Work out the finished part from the listing and answer in its coordinate system (mm). Round coordinates to 2 decimals unless told otherwise and drop trailing zeros. Loops run counter-clockwise (first coordinate to the right, second up) from the corner with the lowest first, then second, coordinate; pieces in that order, holes last. Notation, with made-up numbers: (1, 83.5) - (8, 83.5) arc R15 ccw to (8, 95.5) - close; hole circle Ø7 at (-38, -19.75). An arc over 180 degrees is marked (long way). Answer as CSV lines item,"result". Start each with the question number.
```python
from build123d import *

# Parameters (mm, degrees)
SKETCH1_R           = 1.29
SKETCH1_R_2         = 2
BOSS_EXTRUDE1_DEPTH = 1.5
FILLET1_R           = 2


with BuildPart() as part:
    # Sketch1 → Boss-Extrude1 (new, symmetric)
    with BuildSketch(Plane.XY):
        with BuildLine():
            Line((-9.367496998, 3.5), (30, 3.5))
            ThreePointArc((30, 3.5), (33.5, 0), (30, -3.5))
            Line((30, -3.5), (-9.367496998, -3.5))
            ThreePointArc((-9.367496998, -3.5), (-10, 0), (-9.367496998, 3.5))
        make_face()
        with Locations((-7, 0)):
            Circle(SKETCH1_R, mode=Mode.SUBTRACT)
        with Locations((7, 0)):
            Circle(SKETCH1_R, mode=Mode.SUBTRACT)
        with Locations((30, 0)):
            Circle(SKETCH1_R, mode=Mode.SUBTRACT)
        Circle(SKETCH1_R_2, mode=Mode.SUBTRACT)
    extrude(amount=BOSS_EXTRUDE1_DEPTH, both=True)

    # Fillet1
    fillet1_edges = [part.edges().sort_by_distance(p)[0] for p in [
        (-9.367496998, 3.5, 0),
        (-9.367496998, -3.5, 0),
    ]]
    fillet(fillet1_edges, radius=FILLET1_R)


solid = part.part
```
Item 1: Section A-A, the plane x = 7 is taken. Give the vertices of the cut face in (y, z), and give its area (3 significant figures).
Item 2: Section B-B, the plane z = -0.8 is taken. Give the vertices of the cut face in (x, y) (3 decimals).
Item 3: Determine the mould class of faces 1 (the face through (5.976, -0.785, -0.021)), 2 (the face through (-10, 0, 0)), 3 (the face through (12, 0, -1.5)) for opening direction X: pulls with the +X half, pulls with the -X half, needs draft (parallel to the pull), parting line crosses it, or undercut.
Item 4: Find the intervals of material crossed by L1, parallel to Y at x = -7, z = 0.3; L2, parallel to X at y = -0.75, z = 0.95; L3, parallel to X at y = -1, z = -0.9, in increasing order.
Answer:
1,outline,"(-3.5, -1.5) - (-1.29, -1.5) - (-1.29, 1.5) - (-3.5, 1.5) - close; (1.29, -1.5) - (3.5, -1.5) - (3.5, 1.5) - (1.29, 1.5) - close"
1,area,"13.3 mm²"
2,outline,"(-9.823, -1.875) arc R2 ccw to (-7.858, -3.5) - (30, -3.5) arc R3.5 ccw to (30, 3.5) - (-7.858, 3.5) arc R2 ccw to (-9.823, 1.875) arc R10 ccw to start; hole circle Ø2.58 at (-7, 0); hole circle Ø4 at (0, 0); hole circle Ø2.58 at (7, 0); hole circle Ø2.58 at (30, 0)"
3,face 1,"undercut"
3,face 2,"pulls with the -X half"
3,face 3,"needs draft"
4,L1,"y = -3.5 to -1.29, 1.29 to 3.5"
4,L2,"x = -9.97 to -8.05, -5.95 to -1.85, 1.85 to 5.95, 8.05 to 28.95, 31.05 to 33.42"
4,L3,"x = -9.95 to -7.81, -6.19 to -1.73, 1.73 to 6.19, 7.81 to 29.19, 30.81 to 33.35"
